from build123d import *

# Parameters (mm, degrees)
BOSS_EXTRUDE1_DEPTH = 5
SKETCH2_R           = 2.0675
SKETCH2_W           = 5
SKETCH2_H           = 5
CUT_EXTRUDE1_DEPTH  = 6


with BuildPart() as part:
    # Sketch1 → Boss-Extrude1 (new body)
    with BuildSketch(Plane.XY):
        with BuildLine():
            Line((-32.85, 77.986683936), (32.85, 77.986683936))
            Line((32.85, 77.986683936), (35.403, 82.408609648))
            Line((35.403, 82.408609648), (39.733127019, 79.908609648))
            Line((39.733127019, 79.908609648), (42.286127019, 84.330535359))
            Line((42.286127019, 84.330535359), (37.956, 86.830535359))
            Line((37.956, 86.830535359), (40.509, 91.252461071))
            Line((40.509, 91.252461071), (44.839127019, 88.752461071))
            Line((44.839127019, 88.752461071), (47.392127019, 93.174386783))
            Line((47.392127019, 93.174386783), (43.062, 95.674386783))
            Line((43.062, 95.674386783), (45.615, 100.096312495))
            ThreePointArc((45.615, 100.096312495), (0, 110), (-45.615, 100.096312495))
            Line((-45.615, 100.096312495), (-43.062, 95.674386783))
            Line((-43.062, 95.674386783), (-47.392127019, 93.174386783))
            Line((-47.392127019, 93.174386783), (-44.839127019, 88.752461071))
            Line((-44.839127019, 88.752461071), (-40.509, 91.252461071))
            Line((-40.509, 91.252461071), (-37.956, 86.830535359))
            Line((-37.956, 86.830535359), (-42.286127019, 84.330535359))
            Line((-42.286127019, 84.330535359), (-39.733127019, 79.908609648))
            Line((-39.733127019, 79.908609648), (-35.403, 82.408609648))
            Line((-35.403, 82.408609648), (-32.85, 77.986683936))
        make_face()
    extrude(amount=BOSS_EXTRUDE1_DEPTH)

    # Sketch2 → Cut-Extrude1 (cut, through all)
    with BuildSketch(Plane.XY.offset(5)):
        with Locations((0, 91.897414387)):
            Circle(SKETCH2_R)
        with Locations((18.5, 91.807821113)):
            Rectangle(SKETCH2_W, SKETCH2_H)
        with Locations((-18.5, 91.807821113)):
            Rectangle(SKETCH2_W, SKETCH2_H)
    extrude(amount=-CUT_EXTRUDE1_DEPTH, mode=Mode.SUBTRACT)


solid = part.part
Input: part model. Units: mm. Frame: model coordinates. A direction names the side the tool comes from. Round coordinates to 2 decimals unless told otherwise and drop trailing zeros. Order: outer loops, then holes, each group sorted by start corner. A loop starts at its lowest first (then second) coordinate and runs counter-clockwise, first axis right, second up. Notation, with made-up numbers: (21.25, -0.75) - (55.25, -0.75) arc R23 ccw to (55.25, 17.25) - close; hole circle Ø4 at (58, 73). An arc over 180 degrees is marked (long way). Answer as a JSON object with one key per item and string values. Group by question number.
(1) Cut plane A-A (x = 0). Return loops of the section in (y, z).
(2) Material intervals for probe 1 along Y at (x, z) = (0, 2.95); probe 2 along X at (y, z) = (82, 2.35); probe 3 along X at (y, z) = (92, 2.25), sorted ascending. Write a range as from..to.
(3) Pin query (flat end, axial travel): P1, Ø2.5, axis at x = 18, z = 1.5, coming from the +Y side; P2, Ø1.5, axis at y = 92, z = 0.5, coming from the +X side; P3, Ø2.5, axis at x = -19, z = 3.5, coming from the +Y side. Return the tip coordinate at first contact, or that it passes through.
(4) Cut plane C-C (x = -26.5). Return loops of the section in (y, z).
(5) Cut plane D-D (y = 98). Return loops of the section in (x, z).
(6) Cut plane B-B (z = 1.75). Count the separate pieces of the cut face and the enclosed holes in it, then the cut area to 3 significant figures.
(7) Draft query along Y for faces 1 (the face through (-1, 94, 5)), 2 (the face through (-46.13, 90.99, 2.46)), 3 (the face through (18, 89.308, 3)). Return one class per face: released by +Y, released by -Y, zero draft, split by the parting line, or undercut.
(8) Reachability of faces 4 (the face through (-16, 92, 3)), 5 (the face through (-44.36, 97.92, 2.46)), 6 (the face through (45.257, 94.407, 2.465)), 7 (the face through (34.11, 80.17, 2.46)) from +Z, -Z, +X, -X, +Y, -Y: full face, straight path, thin tool, end or side. Return the list, or none.
Here are the results:
{
 "1": {"outline": "(77.99, 0) - (89.83, 0) - (89.83, 5) - (77.99, 5) - close; (93.96, 0) - (110, 0) - (110, 5) - (93.96, 5) - close"},
 "2": {"probe 1": "y = 77.99..89.83, 93.96..110", "probe 2": "x = -40.94..-36.11, -35.17..35.17, 36.11..40.94", "probe 3": "x = -46.71..-21, -16..-2.06, 2.06..16, 21..46.71"},
 "3": {"P1": "stops at y = 108.72", "P2": "stops at x = 47.15", "P3": "stops at y = 108.56"},
 "4": {"outline": "(77.99, 0) - (106.76, 0) - (106.76, 5) - (77.99, 5) - close"},
 "5": {"outline": "(-44.4, 0) - (44.4, 0) - (44.4, 5) - (-44.4, 5) - close"},
 "6": {"separate pieces": "1", "enclosed holes": "3", "area": "2,380 mm^2"},
 "7": {"face 1": "zero draft", "face 2": "released by -Y", "face 3": "undercut"},
 "8": {"face 4": "+Z, -Z", "face 5": "+Z, -Z, -X", "face 6": "+Z, -Z, +X", "face 7": "+Z, -Z, -Y"}
}
